Model file for the job. Use its own axes, mm. A direction names the side the tool comes from. Coordinates: 2 decimals unless noted, no trailing zeros. Order: outer loops, then holes, each group sorted by start corner. A loop starts at its lowest first (then second) coordinate and runs counter-clockwise, first axis right, second up. Notation, with made-up numbers: (25, 65) -> (45, 65) arc R24 cw to (45, 88) -> close; hole circle Ø6 at (66.5, 12). An arc over 180 degrees is marked (long way). Return JSON: item names as keys, results as strings. Group by question number.
1) Probe line 1 (Z direction, x = 198.5, y = -41); line 2 (Y direction, x = 21, z = 18.5); line 3 (X direction, y = -36, z = 59). List the from-to ranges inside material, lowest first.
2) Cut at B-B (y = -46.5). Write the cut outline in (x, z).
3) Pull direction Y, two halves, no side cores. Call faces 4 (the flat face through (111, 0, 41)), 5 (the flat face through (109, -27, 80)), 6 (the flat face through (0, -52, 39)): +Y half, -Y half, draft (parallel to the pull), parting line (faces both ways), or undercut.
4) Which spindle directions (+Z, -Z, +X, -X, +Y, -Y) get a long thin tool onto all of the face, cutting with end or side? Do faces 1 (the flat face through (109, -27, 4)), 2 (the cylindrical face through (216.394, -2.028, 69.069)), 3 (the flat face through (111, -27, 0)). Say none if no direction does.
5) Cut at D-D (x = 112.5). Write the cut outline in (y, z), and give its area (3 significant figures).
6) Cut at C-C (z = 63). Write the cut outline in (x, y), and give its area (3 significant figures).
7) Cut at A-A (z = 14.5). Write the cut outline in (x, y), and give its area (3 significant figures).
8) Flat gauge pin, fed straight in: pin 1 (4 mm diameter, centred on x = 154, y = -27.5, fed in from -Z). Where does the tip first touch, or does it go through?
from build123d import *

# Parameters (mm, degrees)
SKETCH1_W           = 225
SKETCH1_H           = 55
BOSS_EXTRUDE1_DEPTH = 84
SHELL1_T            = -4
SKETCH2_R           = 2
CUT_EXTRUDE1_DEPTH  = 246.523929587


with BuildPart() as part:
    # Sketch1 → Boss-Extrude1 (new body)
    with BuildSketch(Plane.XY):
        with Locations((112.5, -27.5)):
            Rectangle(SKETCH1_W, SKETCH1_H)
    extrude(amount=BOSS_EXTRUDE1_DEPTH)

    # Shell1
    shell1_openings = [part.faces().sort_by_distance(p)[0] for p in [
        (0, -27.5, 42),
    ]]
    offset(amount=SHELL1_T, openings=shell1_openings, kind=Kind.INTERSECTION)

    # Sketch2 → Cut-Extrude1 (cut, through all)
    with BuildSketch(Plane.XZ.offset(4)):
        with Locations(Location((14.707468467, 70.14380551, 0), (0, 0, 270))):
            Circle(SKETCH2_R)
        with Locations(Location((14.707468467, 14.5, 0), (0, 0, 270))):
            Circle(SKETCH2_R)
        with Locations(Location((214.707468467, 70.14380551, 0), (0, 0, 270))):
            Circle(SKETCH2_R)
        with Locations(Location((214.707468467, 14.5, 0), (0, 0, 270))):
            Circle(SKETCH2_R)
    extrude(amount=-CUT_EXTRUDE1_DEPTH, mode=Mode.SUBTRACT)


solid = part.part
Answers below:
{
 "1": {"line 1": "z = 0 to 4, 80 to 84", "line 2": "y = -55 to -51, -4 to 0", "line 3": "x = 221 to 225"},
 "2": {"outline": "(0, 0) -> (225, 0) -> (225, 84) -> (0, 84) -> (0, 80) -> (221, 80) -> (221, 4) -> (0, 4) -> close"},
 "3": {"face 4": "+Y half", "face 5": "undercut", "face 6": "draft"},
 "4": {"face 1": "-X", "face 2": "+Y", "face 3": "-Z, +X, -X, +Y, -Y"},
 "5": {"outline": "(-55, 0) -> (0, 0) -> (0, 84) -> (-55, 84) -> close; hole (-51, 4) -> (-4, 4) -> (-4, 80) -> (-51, 80) -> close", "area": "1,050 mm^2"},
 "6": {"outline": "(0, -55) -> (225, -55) -> (225, 0) -> (0, 0) -> (0, -4) -> (221, -4) -> (221, -51) -> (0, -51) -> close", "area": "1,990 mm^2"},
 "7": {"outline": "(0, -55) -> (225, -55) -> (225, 0) -> (216.71, 0) -> (216.71, -4) -> (221, -4) -> (221, -51) -> (0, -51) -> close; (0, -4) -> (12.71, -4) -> (12.71, 0) -> (0, 0) -> close; (16.71, -4) -> (212.71, -4) -> (212.71, 0) -> (16.71, 0) -> close", "area": "1,960 mm^2"},
 "8": {"pin 1": "stops at z = 0"}
}
